```python
from build123d import *

# Parameters (mm, degrees)
SKETCH_2_R                   = 4
SKETCH_2_R_2                 = 1.75
EXTRUDE_1_DEPTH              = 5.6
PATTERN_LINEAR_1_COUNT       = 3
PATTERN_LINEAR_1_PITCH       = 12.5
EXTRUDE_2_DEPTH              = 6.25
EXTRUDE_2_DEPTH_BACK         = 37.25
SKETCH_3_W                   = 25
SKETCH_3_H                   = 2.5
SKETCH_4_R                   = 5.5
CUT_EXTRUDE_1_DEPTH          = 6.9
PATTERN_LINEAR_2_COUNT       = 4
PATTERN_LINEAR_2_PITCH       = 12.5
PATTERN_LINEAR_4_COUNT       = 2
PATTERN_LINEAR_4_PITCH       = 12.5
PATTERN_START                = 12.5
PATTERN_LINEAR_3_OUTLINE_R   = 1.75
PATTERN_LINEAR_3_DEPTH       = 5.6
PATTERN_START_2              = 25
PATTERN_LINEAR_3_2_OUTLINE_R = 1.75
PATTERN_LINEAR_3_2_DEPTH     = 5.6
MIRROR_3_COPY_1_SKETCH_R     = 5.5
MIRROR_3_COPY_1_DEPTH        = 6.9
MIRROR_3_COPY_2_SKETCH_R     = 5.5
MIRROR_3_COPY_2_DEPTH        = 6.9
MIRROR_3_COPY_3_SKETCH_R     = 5.5
MIRROR_3_COPY_3_DEPTH        = 6.9
MIRROR_3_COPY_4_SKETCH_R     = 5.5
MIRROR_3_COPY_4_DEPTH        = 6.9
SKETCH_5_W                   = 3
SKETCH_5_H                   = 10
EXTRUDE_3_DEPTH              = 5.6
EXTRUDE_4_DEPTH              = 25
EXTRUDE_4_DEPTH_BACK         = 6
SKETCH_6_R                   = 4
SKETCH_7_W                   = 20
SKETCH_7_H                   = 7
EXTRUDE_5_DEPTH              = 10
SKETCH_8_W                   = 5
SKETCH_8_H                   = 7
CUT_EXTRUDE_2_DEPTH          = 10
SKETCH_12_W                  = 25.926545396
SKETCH_12_H                  = 6.65
SKETCH_12_W_2                = 26.106427018
SKETCH_12_H_2                = 6.25
CUT_EXTRUDE_5_DEPTH          = 10
CUT_EXTRUDE_6_DEPTH          = 3.4
CUT_EXTRUDE_6_DEPTH_BACK     = 3.4
SKETCH_13_R                  = 4
SKETCH_14_R                  = 1.6
CUT_EXTRUDE_7_DEPTH          = 56.2


# Read off the part's stored shape, not the designer's step: the pattern linear step
with BuildPart() as part:
    # Sketch 2 → Extrude 1 (new body)
    with BuildSketch(Plane.XY):
        Circle(SKETCH_2_R)
        Circle(SKETCH_2_R_2, mode=Mode.SUBTRACT)
    extrude_1 = extrude(amount=EXTRUDE_1_DEPTH)


with BuildPart() as pattern_linear_1_1:
    # Pattern Linear 1: pattern copy
    add(part.part.moved(Location(Vector(0, 0, 1) * (1 * PATTERN_LINEAR_1_PITCH))))


with BuildPart() as pattern_linear_1_2:
    # Pattern Linear 1: pattern copy
    add(part.part.moved(Location(Vector(0, 0, 1) * (2 * PATTERN_LINEAR_1_PITCH))))


with BuildPart() as part_1:
    add(part.part)

    add(pattern_linear_1_1.part)  # Extrude 2 merges Pattern Linear 1_1

    add(pattern_linear_1_2.part)  # Extrude 2 merges Pattern Linear 1_2
    # Sketch 3 → Extrude 2 (add, two sides: drawn at the far end of the back side and taken through both)
    with BuildSketch(Plane(origin=(0, 0, 0), x_dir=(-1, 0, 0), z_dir=(0, 0, -1)).offset(-EXTRUDE_2_DEPTH_BACK)):
        with Locations((16.299671038, 0)):
            Rectangle(SKETCH_3_W, SKETCH_3_H)
    extrude(amount=EXTRUDE_2_DEPTH + EXTRUDE_2_DEPTH_BACK)

    # Sketch 4 → Cut-Extrude 1 (cut)
    with BuildSketch(Plane.XY.offset(5.6)):
        Circle(SKETCH_4_R)
    cut_extrude_1 = extrude(amount=CUT_EXTRUDE_1_DEPTH, mode=Mode.SUBTRACT)

    # Pattern Linear 2: Cut-Extrude 1 ×4
    with Locations(*[(0, 0, i * PATTERN_LINEAR_2_PITCH) for i in range(1, PATTERN_LINEAR_2_COUNT)]):
        add(cut_extrude_1, mode=Mode.SUBTRACT)

    # Pattern Linear 4: Cut-Extrude 1 ×2
    with Locations(*[(0, 0, -i * PATTERN_LINEAR_4_PITCH) for i in range(1, PATTERN_LINEAR_4_COUNT)]):
        add(cut_extrude_1, mode=Mode.SUBTRACT)

    # Mirror 1: Extrude 1 across plane
    add(extrude_1.mirror(Plane.ZY.offset(16.299671038)))

    # Pattern Linear 3 outline → Pattern Linear 3 (add)
    with BuildSketch(Plane.XY.offset(PATTERN_START)):
        with BuildLine():
            ThreePointArc((-28.799671038, 1.25), (-36.599342077, 0), (-28.799671038, -1.25))
            Line((-28.799671038, -1.25), (-28.799671038, 1.25))
        make_face()
        with Locations((-32.599342077, 0)):
            Circle(PATTERN_LINEAR_3_OUTLINE_R, mode=Mode.SUBTRACT)
    extrude(amount=PATTERN_LINEAR_3_DEPTH)

    # Pattern Linear 3 2 outline → Pattern Linear 3 2 (add)
    with BuildSketch(Plane.XY.offset(PATTERN_START_2)):
        with BuildLine():
            ThreePointArc((-28.799671038, 1.25), (-36.599342077, 0), (-28.799671038, -1.25))
            Line((-28.799671038, -1.25), (-28.799671038, 1.25))
        make_face()
        with Locations((-32.599342077, 0)):
            Circle(PATTERN_LINEAR_3_2_OUTLINE_R, mode=Mode.SUBTRACT)
    extrude(amount=PATTERN_LINEAR_3_2_DEPTH)

    # Mirror 3: Cut-Extrude 1 across plane
    add(cut_extrude_1.mirror(Plane.ZY.offset(16.299671038)), mode=Mode.SUBTRACT)

    # Mirror 3 copy 1 sketch → Mirror 3 copy 1 (cut)
    with BuildSketch(Plane(origin=(-32.599342077, 0, 18.1), x_dir=(-1, 0, 0), z_dir=(0, 0, 1))):
        Circle(MIRROR_3_COPY_1_SKETCH_R)
    extrude(amount=MIRROR_3_COPY_1_DEPTH, mode=Mode.SUBTRACT)

    # Mirror 3 copy 2 sketch → Mirror 3 copy 2 (cut)
    with BuildSketch(Plane(origin=(-32.599342077, 0, 30.6), x_dir=(-1, 0, 0), z_dir=(0, 0, 1))):
        Circle(MIRROR_3_COPY_2_SKETCH_R)
    extrude(amount=MIRROR_3_COPY_2_DEPTH, mode=Mode.SUBTRACT)

    # Mirror 3 copy 3 sketch → Mirror 3 copy 3 (cut)
    with BuildSketch(Plane(origin=(-32.599342077, 0, 43.1), x_dir=(-1, 0, 0), z_dir=(0, 0, 1))):
        Circle(MIRROR_3_COPY_3_SKETCH_R)
    extrude(amount=MIRROR_3_COPY_3_DEPTH, mode=Mode.SUBTRACT)

    # Mirror 3 copy 4 sketch → Mirror 3 copy 4 (cut)
    with BuildSketch(Plane(origin=(-32.599342077, 0, -6.9), x_dir=(-1, 0, 0), z_dir=(0, 0, 1))):
        Circle(MIRROR_3_COPY_4_SKETCH_R)
    extrude(amount=MIRROR_3_COPY_4_DEPTH, mode=Mode.SUBTRACT)

    # Sketch 5 → Extrude 3 (add)
    with BuildSketch(Plane(origin=(0, 0, 0), x_dir=(-1, 0, 0), z_dir=(0, 0, -1))):
        with Locations((32.599342077, 8.708099244)):
            Rectangle(SKETCH_5_W, SKETCH_5_H)
    extrude_3 = extrude(amount=-EXTRUDE_3_DEPTH)

    # Mirror 4: Extrude 3 across plane
    add(extrude_3.mirror(Plane(origin=(0, 0, 15.3), x_dir=(1, 0, 0), z_dir=(0, 0, -1))))

    # Sketch 6 → Extrude 4 (add, two sides: drawn at the far end of the back side and taken through both)
    with BuildSketch(Plane(origin=(0, 0, 25), x_dir=(-1, 0, 0), z_dir=(0, 0, -1)).offset(-EXTRUDE_4_DEPTH_BACK)):
        with Locations((32.599342077, 13.708099244)):
            Circle(SKETCH_6_R)
    extrude(amount=EXTRUDE_4_DEPTH + EXTRUDE_4_DEPTH_BACK)

    # Sketch 7 → Extrude 5 (add)
    with BuildSketch(Plane(origin=(0, 1.25, 0), x_dir=(1, 0, 0), z_dir=(0, 1, 0))):
        with Locations((-17.243270755, -15.3)):
            Rectangle(SKETCH_7_W, SKETCH_7_H)
    extrude(amount=EXTRUDE_5_DEPTH)

    # Sketch 8 → Cut-Extrude 2 (cut)
    with BuildSketch(Plane(origin=(0, 0, 11.8), x_dir=(-1, 0, 0), z_dir=(0, 0, -1))):
        Polygon((6.030917846, 10.25), (20.326387044, 9.963182504), (20.326387044, 1.25), (27.243270755, 1.25), (30.785730431, 14.859314756), (3.995086375, 15.396829498), align=None)
        with Locations((12.743270755, 4.75)):
            Rectangle(SKETCH_8_W, SKETCH_8_H)
    extrude(amount=-CUT_EXTRUDE_2_DEPTH, mode=Mode.SUBTRACT)

    # Sketch 12 → Cut-Extrude 5 (cut)
    with BuildSketch(Plane(origin=(0, 1.25, 0), x_dir=(1, 0, 0), z_dir=(0, 1, 0))):
        with Locations((-16.867780953, -33.925)):
            Rectangle(SKETCH_12_W, SKETCH_12_H)
        with Locations((-16.852884547, 3.125)):
            Rectangle(SKETCH_12_W_2, SKETCH_12_H_2)
    extrude(amount=-CUT_EXTRUDE_5_DEPTH, mode=Mode.SUBTRACT)

    # Sketch 13 → Cut-Extrude 6 (cut, two sides: drawn at the far end of the back side and taken through both)
    with BuildSketch(Plane(origin=(0, 0, 15.3), x_dir=(-1, 0, 0), z_dir=(0, 0, -1)).offset(-CUT_EXTRUDE_6_DEPTH_BACK)):
        with Locations((32.599342077, 13.708099244)):
            Circle(SKETCH_13_R)
    extrude(amount=CUT_EXTRUDE_6_DEPTH + CUT_EXTRUDE_6_DEPTH_BACK, mode=Mode.SUBTRACT)

    # Sketch 14 → Cut-Extrude 7 (cut)
    with BuildSketch(Plane(origin=(0, 0, 0), x_dir=(-1, 0, 0), z_dir=(0, 0, -1))):
        with Locations((32.599342077, 13.708099244)):
            Circle(SKETCH_14_R)
    extrude(amount=-CUT_EXTRUDE_7_DEPTH, mode=Mode.SUBTRACT)

    # Chamfer 1
    # the kernel refuses this chamfer: 1.81151278, 1 mm, written as the material it adds along each edge
    with BuildSketch(Plane(origin=(-31.099342077, 3.708099244, 0), x_dir=(0.8415361936638334, -0.540200735610187, 0), z_dir=(0, 0, 1))) as chamfer_1_piece_1:
        with BuildLine():
            Line((1.429397457, 0), (-0.413759333, 0.557495143))
            Line((-0.413759333, 0.557495143), (-0.444248404, 0.537923532))
            ThreePointArc((-0.444248404, 0.537923532), (-0.217578261, 0.271879907), (-0.030489071, -0.019571611))
            Line((-0.030489071, -0.019571611), (0.006709967, -0.03560348))
            ThreePointArc((0.006709967, -0.03560348), (0.714480275, 0.032881444), (1.423788773, -0.035793492))
            Line((1.423788773, -0.035793492), (1.429397457, 0))
        make_face()
    extrude(amount=5.6)
    with BuildSketch(Plane(origin=(-34.099342077, 3.708099244, 0), x_dir=(-0.8415361936638353, -0.5402007356101841, 0), z_dir=(0, 0, 1))) as chamfer_1_piece_2:
        with BuildLine():
            Line((1.429397457, 0), (-0.413759333, -0.557495143))
            Line((-0.413759333, -0.557495143), (-0.444248404, -0.537923532))
            ThreePointArc((-0.444248404, -0.537923532), (-0.217578261, -0.271879907), (-0.030489071, 0.019571611))
            Line((-0.030489071, 0.019571611), (0.006709967, 0.03560348))
            ThreePointArc((0.006709967, 0.03560348), (0.714480275, -0.032881444), (1.423788773, 0.035793492))
            Line((1.423788773, 0.035793492), (1.429397457, 0))
        make_face()
    extrude(amount=5.6)
    with BuildSketch(Plane(origin=(-31.099342077, 3.708099244, 30.6), x_dir=(0.8415361938100423, -0.5402007353824197, 0), z_dir=(0, 0, -1))) as chamfer_1_piece_3:
        with BuildLine():
            Line((1.429397457, 0), (-0.413759333, -0.557495144))
            Line((-0.413759333, -0.557495144), (-0.444248404, -0.537923533))
            ThreePointArc((-0.444248404, -0.537923533), (-0.217578261, -0.271879907), (-0.030489071, 0.019571611))
            Line((-0.030489071, 0.019571611), (0.006709967, 0.03560348))
            ThreePointArc((0.006709967, 0.03560348), (0.714480275, -0.032881444), (1.423788773, 0.035793492))
            Line((1.423788773, 0.035793492), (1.429397457, 0))
        make_face()
    extrude(amount=5.6)
    with BuildSketch(Plane(origin=(-34.099342077, 3.708099244, 30.6), x_dir=(-0.8415361937600511, -0.5402007354602969, 0), z_dir=(0, 0, -1))) as chamfer_1_piece_4:
        with BuildLine():
            Line((1.429397457, 0), (-0.413759333, 0.557495144))
            Line((-0.413759333, 0.557495144), (-0.444248404, 0.537923533))
            ThreePointArc((-0.444248404, 0.537923533), (-0.217578261, 0.271879907), (-0.030489071, -0.019571611))
            Line((-0.030489071, -0.019571611), (0.006709967, -0.03560348))
            ThreePointArc((0.006709967, -0.03560348), (0.714480275, 0.032881444), (1.423788773, -0.035793492))
            Line((1.423788773, -0.035793492), (1.429397457, 0))
        make_face()
    extrude(amount=5.6)


solid = part_1.part
```
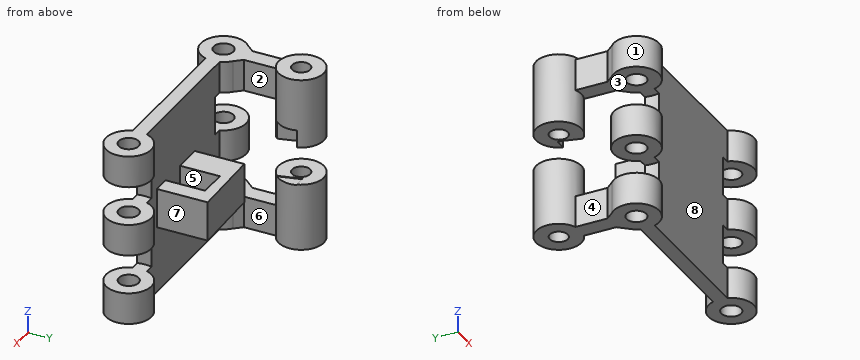
Build history of the part. All positions in model axes, mm. Face numbers are marked on the shaded views. A direction names the side the tool comes from. Give positions to 0.01 mm unless a question says otherwise; leave off trailing zeros. Order: outer loops, then holes, each group sorted by start corner. A loop starts at its lowest first (then second) coordinate and runs counter-clockwise, first axis right, second up. Notation, with made-up numbers: M 2,63 L 38,63 A20 ccw 38,96 Z; hole C 2,-10.5 d7. An arc over 180 degrees is marked long. Write item = value, one per line. Start each with the question number.
(1) Slice it at B-B on x = 0. Write the cut outline in (y, z).
(2) Probe L1, parallel to Z at x = -29, y = 0; L2, parallel to Y at x = 0, z = 4.35; L3, parallel to X at y = 6.5, z = 18. List the from-to ranges inside material, lowest first. Write a range as [from, to].
(3) Which spindle directions (+Z, -Z, +X, -X, +Y, -Y) get a long thin tool onto all of the face, cutting with end or side? Do the marked faces 4, 5, 6, 7 and 8. Say none if no direction does.
(4) Slice it at C-C on z = 15. Write the cut outline in (x, y), plus the area to 3 significant figures.
(5) Slice it at A-A on y = 9. Write the cut outline in (x, z).
(6) Slice it at D-D on y = 16. Write the cut outline in (x, z), plus the area to 3 significant figures.
(7) Pin check, flat tips, straight feed: pin 1 Ø8 at (y, z) = (5, 8.5) entering from -X; pin 2 Ø6 at (x, y) = (-1.5, 9) entering from +Z; pin 3 Ø4.5 at (x, y) = (-15, 4) entering from -Z; pin 4 Ø7.5 at (x, z) = (-21.5, 8) entering from -Y. Stop position of each tip, or through.
(8) Two-plate mould, pull along X, no slides. Class the marked faces 1, 2 and 3: released by +X, released by -X, zero draft, split by the parting line, or undercut.
Responses:
q1.outline = M -4,0 L -1.75,0 L -1.75,5.6 L -4,5.6 Z; M -4,12.5 L -1.75,12.5 L -1.75,18.1 L -4,18.1 Z; M -4,25 L -1.75,25 L -1.75,30.6 L -4,30.6 Z; M 1.75,0 L 4,0 L 4,5.6 L 1.75,5.6 Z; M 1.75,12.5 L 4,12.5 L 4,18.1 L 1.75,18.1 Z; M 1.75,25 L 4,25 L 4,30.6 L 1.75,30.6 Z
q2.L1 = [0, 5.6], [12.5, 18.1], [25, 30.6]
q2.L2 = [-4, -1.75], [1.75, 4]
q2.L3 = [-20.33, -15.24], [-10.24, -7.24]
q3.face_4 = +Z, -Z, -X
q3.face_5 = +Z, -Z
q3.face_6 = +Z, -Z, +X
q3.face_7 = +Z, -Z, +Y
q3.face_8 = +Z, -Z, -Y
q4.outline = M -28.8,-1.25 L -3.8,-1.25 A4 ccw long -3.8,1.25 L -7.24,1.25 L -7.24,10.23 L -20.33,9.96 L -20.33,1.25 L -28.8,1.25 A4 ccw long Z; hole C -32.6,0 d3.5; hole M -15.24,1.25 L -10.24,1.25 L -10.24,8.25 L -15.24,8.25 Z; hole C 0,0 d3.5
q4.area = 224 mm2
q5.outline = M -34.1,0 L -31.1,0 L -31.1,5.6 L -34.1,5.6 Z; M -34.1,25 L -31.1,25 L -31.1,30.6 L -34.1,30.6 Z; M -20.33,11.8 L -7.24,11.8 L -7.24,18.8 L -20.33,18.8 Z
q6.outline = M -35.88,0 L -29.32,0 L -29.32,11.9 L -35.88,11.9 Z; M -35.88,18.7 L -29.32,18.7 L -29.32,31 L -35.88,31 Z
q6.area = 159 mm2
q7.pin_1 = -35.91
q7.pin_2 = through
q7.pin_3 = 11.8
q7.pin_4 = -1.25
q8.face_1 = undercut
q8.face_2 = released by +X
q8.face_3 = zero draft
